Print and shaded views of the part. All mm, measured from the part's lowest x, y and z. A direction names the side the tool comes from. Coordinates: 2 decimals unless noted, no trailing zeros. Order: outer loops, then holes, each group sorted by start corner. A loop starts at its lowest first (then second) coordinate and runs counter-clockwise, first axis right, second up. Notation, with made-up numbers: (30, 18) -> (47, 18) arc R7 cw to (47, 30) -> close; hole circle Ø8 at (60, 33.25). An arc over 180 degrees is marked (long way). Write item = value, one per line. Start each with the question number.
Q1. Mould opens along X. For the marked faces 3, 4 and 5 say: +X half, -X half, draft (parallel to the pull), parting line (faces both ways), or undercut.
Q2. Flat gauge pins, fed straight in: pin 1 (12 mm diameter, centred on x = 21.5, z = 11.5, fed in from +Y); pin 2 (6.5 mm diameter, centred on x = 58, y = 58, fed in from +Z); pin 3 (1.5 mm diameter, centred on x = 34.5, z = 22, fed in from +Y). Where does each tip first touch, or does it go through?
Q3. Wall check: line 1 (Y direction, x = 58, z = 2.1); line 2 (Y direction, x = 8, z = 2.2); line 3 (X direction, y = 8.5, z = 6). Give the ranges that are in metal, low to high. Write a range as from..to.
Q4. Cut at A-A, the plane x = 8. List the corners of the cut face in (y, z), plus the area to 3 significant figures.
Q5. Cut at C-C, the plane y = 28. List the corners of the cut face in (x, z).
Q6. Cut at B-B, the plane z = 12.25. List the corners of the cut face in (x, y), plus the area to 3 significant figures.
Q7. 3-axis set-ups, long thin cutter, end or side, ignore diameter. For the marked faces 1 and 2: which of +Z, -Z, +X, -X, +Y, -Y reach the whole face in a straight line?
Q8. Cut at D-D, the plane x = 16. List the corners of the cut face in (y, z), plus the area to 3 significant figures.
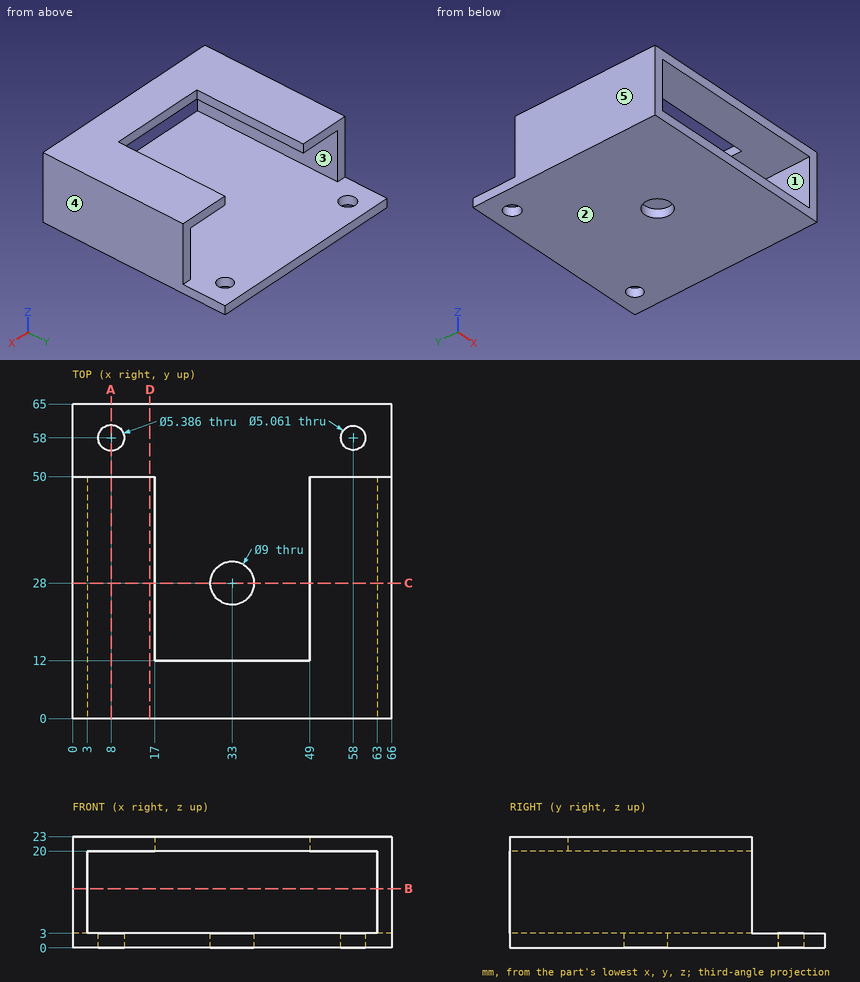
Here are the results:
q1.face_3 = undercut
q1.face_4 = +X half
q1.face_5 = -X half
q2.pin_1 = through
q2.pin_2 = 3
q2.pin_3 = 12
q3.line_1 = 0..55.47, 60.53..65
q3.line_2 = 0..55.31, 60.69..65
q3.line_3 = 0..3, 63..66
q4.outline = (0, 0) -> (55.31, 0) -> (55.31, 3) -> (0, 3) -> close; (0, 20) -> (50, 20) -> (50, 23) -> (0, 23) -> close; (60.69, 0) -> (65, 0) -> (65, 3) -> (60.69, 3) -> close
q4.area = 329 mm²
q5.outline = (0, 0) -> (28.5, 0) -> (28.5, 3) -> (3, 3) -> (3, 20) -> (17, 20) -> (17, 23) -> (0, 23) -> close; (37.5, 0) -> (66, 0) -> (66, 23) -> (49, 23) -> (49, 20) -> (63, 20) -> (63, 3) -> (37.5, 3) -> close
q6.outline = (0, 0) -> (3, 0) -> (3, 50) -> (0, 50) -> close; (63, 0) -> (66, 0) -> (66, 50) -> (63, 50) -> close
q6.area = 300 mm²
q7.face_1 = +Y, -Y
q7.face_2 = -Z, +X, -X, +Y, -Y
q8.outline = (0, 0) -> (65, 0) -> (65, 3) -> (0, 3) -> close; (0, 20) -> (50, 20) -> (50, 23) -> (0, 23) -> close
q8.area = 345 mm²
